CAD build for the part. Positions are in the model's coordinates, mm. A direction names the side the tool comes from. Coordinates: 2 decimals unless noted, no trailing zeros. Loops run counter-clockwise (first coordinate to the right, second up) from the corner with the lowest first, then second, coordinate; pieces in that order, holes last. Notation, with made-up numbers: (-20, 16) -> (5, 16) arc R20 cw to (5, 35) -> close; hole circle Ø8 at (17.5, 18). An arc over 180 degrees is marked (long way). Answer as a JSON object with one key per item and string values. Group by question number.
from build123d import *

# Parameters (mm, degrees)
SKETCH1_W            = 63.5
SKETCH1_H            = 33.401
SKETCH1_W_2          = 10.16
SKETCH1_H_2          = 3.175
SKETCH1_W_3          = 40.64
SKETCH1_H_3          = 20.066
MAIN_EXTRUSION_DEPTH = 3.175
SKETCH3_R            = 2.2225
MOUNTING_HOLES_DEPTH = 37.777630008
TAB_CUTOUT_DEPTH     = 37.777630008
FILLET1_R            = 5.08
SKETCH6_W            = 69.522251557
SKETCH6_H            = 29.320751893
CUT_EXTRUDE3_DEPTH   = 37.777630008


with BuildPart() as part:
    # Sketch1 → Main Extrusion (new body)
    with BuildSketch(Plane(origin=(0, 0, 0), x_dir=(1, 0, 0), z_dir=(0, 1, 0))):
        with Locations((0, 1.5875)):
            Rectangle(SKETCH1_W, SKETCH1_H)
        with Locations((21.59, 14.1605)):
            Rectangle(SKETCH1_W_2, SKETCH1_H_2, mode=Mode.SUBTRACT)
        with Locations((1.27, 14.1605)):
            Rectangle(SKETCH1_W_2, SKETCH1_H_2, mode=Mode.SUBTRACT)
        with Locations((-19.05, 14.1605)):
            Rectangle(SKETCH1_W_2, SKETCH1_H_2, mode=Mode.SUBTRACT)
        Rectangle(SKETCH1_W_3, SKETCH1_H_3, mode=Mode.SUBTRACT)
    extrude(amount=MAIN_EXTRUSION_DEPTH)

    # Sketch3 → Mounting Holes (cut, through all)
    with BuildSketch(Plane(origin=(0, 3.175, 0), x_dir=(1, 0, 0), z_dir=(0, 1, 0))):
        with Locations(Location((-24.992246486, 4.9657, 0), (0, 0, 270))):
            Circle(SKETCH3_R)
        with Locations(Location((-24.992246486, -4.9657, 0), (0, 0, 270))):
            Circle(SKETCH3_R)
        with Locations(Location((24.992246486, -4.9657, 0), (0, 0, 90))):
            Circle(SKETCH3_R)
        with Locations(Location((24.992246486, 4.9657, 0), (0, 0, 90))):
            Circle(SKETCH3_R)
    extrude(amount=-MOUNTING_HOLES_DEPTH, mode=Mode.SUBTRACT)

    # Sketch5 → Tab cutout (cut, through all)
    with BuildSketch(Plane(origin=(0, 3.175, 0), x_dir=(1, 0, 0), z_dir=(0, 1, 0))):
        Polygon((-20.32, 0), (-20.32, 0.889), (-27.305, 0.889), (-27.305, -0.889), (-20.32, -0.889), align=None)
        Polygon((27.305, -0.889), (20.32, -0.889), (20.32, 0), (20.32, 0.889), (27.305, 0.889), align=None)
    extrude(amount=-TAB_CUTOUT_DEPTH, mode=Mode.SUBTRACT)

    # Fillet1
    fillet1_edges = [part.edges().sort_by_distance(p)[0] for p in [
        (31.75, 1.5875, 15.113),
        (-31.75, 1.5875, 15.113),
        (-31.75, 1.5875, -18.288),
        (31.75, 1.5875, -18.288),
    ]]
    fillet(fillet1_edges, radius=FILLET1_R)

    # Sketch6 → Cut-Extrude3 (cut, through all)
    with BuildSketch(Plane(origin=(0, 3.175, 0), x_dir=(1, 0, 0), z_dir=(0, 1, 0))):
        with Locations((-0.129688159, -3.818782995)):
            Rectangle(SKETCH6_W, SKETCH6_H)
    extrude(amount=-CUT_EXTRUDE3_DEPTH, mode=Mode.SUBTRACT)


solid = part.part
Item 1: 3-axis set-ups, long thin cutter, end or side, ignore diameter. For faces 5 (the flat face through (1, 2, -12.573)), 6 (the cylindrical face through (30.22, 1.61, -16.84)): which of +Z, -Z, +X, -X, +Y, -Y reach the whole face in a straight line?
Item 2: Band-saw the part on D-D, the plane z = -17. List the corners of the cut face in (x, y) (3 decimals).
Item 3: Band-saw the part on A-A, the plane x = -16.5. List the corners of the cut face in (y, z) (3 decimals).
Item 4: Pull direction X, two halves, no side cores. Call faces 1 (the flat face through (31.75, 2, -12)), 2 (the flat face through (0, 2, -10.842)), 3 (the cylindrical face through (-30.3, 1.61, -16.76)), 4 (the flat face through (-19, 2, -12.573)): +X half, -X half, draft (parallel to the pull), parting line (faces both ways), or undercut.
Item 5: Band-saw the part on B-B, the plane z = -14.25. List the corners of the cut face in (x, y) (3 decimals), and give its area (3 significant figures).
Item 6: Drill centre lines: L1, parallel to X at y = 2.7, z = -12.75; L2, parallel to Z at x = 2, y = 1.9; L3, parallel to X at y = 0.75, z = -14.5. Where is each one in solid material? Low to high.
Item 7: Band-saw the part on C-C, the plane y = 0.95. List the corners of the cut face in (x, z).
Reply:
{
 "1": {"face 5": "+Y, -Y", "face 6": "-Z, +X, +Y, -Y"},
 "2": {"outline": "(-30.05, 0) -> (30.05, 0) -> (30.05, 3.175) -> (-30.05, 3.175) -> close"},
 "3": {"outline": "(0, -18.288) -> (3.175, -18.288) -> (3.175, -15.748) -> (0, -15.748) -> close; (0, -12.573) -> (3.175, -12.573) -> (3.175, -10.842) -> (0, -10.842) -> close"},
 "4": {"face 1": "+X half", "face 2": "draft", "face 3": "-X half", "face 4": "undercut"},
 "5": {"outline": "(-31.642, 0) -> (-24.13, 0) -> (-24.13, 3.175) -> (-31.642, 3.175) -> close; (-13.97, 0) -> (-3.81, 0) -> (-3.81, 3.175) -> (-13.97, 3.175) -> close; (6.35, 0) -> (16.51, 0) -> (16.51, 3.175) -> (6.35, 3.175) -> close; (26.67, 0) -> (31.642, 0) -> (31.642, 3.175) -> (26.67, 3.175) -> close", "area": "104 mm²"},
 "6": {"L1": "-31.75 to -24.13, -13.97 to -3.81, 6.35 to 16.51, 26.67 to 31.75", "L2": "-18.29 to -15.75, -12.57 to -10.84", "L3": "-31.58 to -24.13, -13.97 to -3.81, 6.35 to 16.51, 26.67 to 31.58"},
 "7": {"outline": "(-31.75, -13.21) arc R5.08 ccw to (-26.67, -18.29) -> (26.67, -18.29) arc R5.08 ccw to (31.75, -13.21) -> (31.75, -10.84) -> (-31.75, -10.84) -> close; hole (-24.13, -15.75) -> (-13.97, -15.75) -> (-13.97, -12.57) -> (-24.13, -12.57) -> close; hole (-3.81, -15.75) -> (6.35, -15.75) -> (6.35, -12.57) -> (-3.81, -12.57) -> close; hole (16.51, -15.75) -> (26.67, -15.75) -> (26.67, -12.57) -> (16.51, -12.57) -> close"}
}
